For this review, use the dimensioned drawing (mm, ordinates from the lowest corner) and the shaded views. Coordinates: 2 decimals unless noted, no trailing zeros. Loops run counter-clockwise (first coordinate to the right, second up) from the corner with the lowest first, then second, coordinate; pieces in that order, holes last. Notation, with made-up numbers: (84, -2) - (95, -2) arc R19 cw to (95, 25) - close; hole circle Ø9 at (29, 16). An arc over 180 degrees is marked (long way). Return JSON: item names as keys, results as strings. Group by question number.
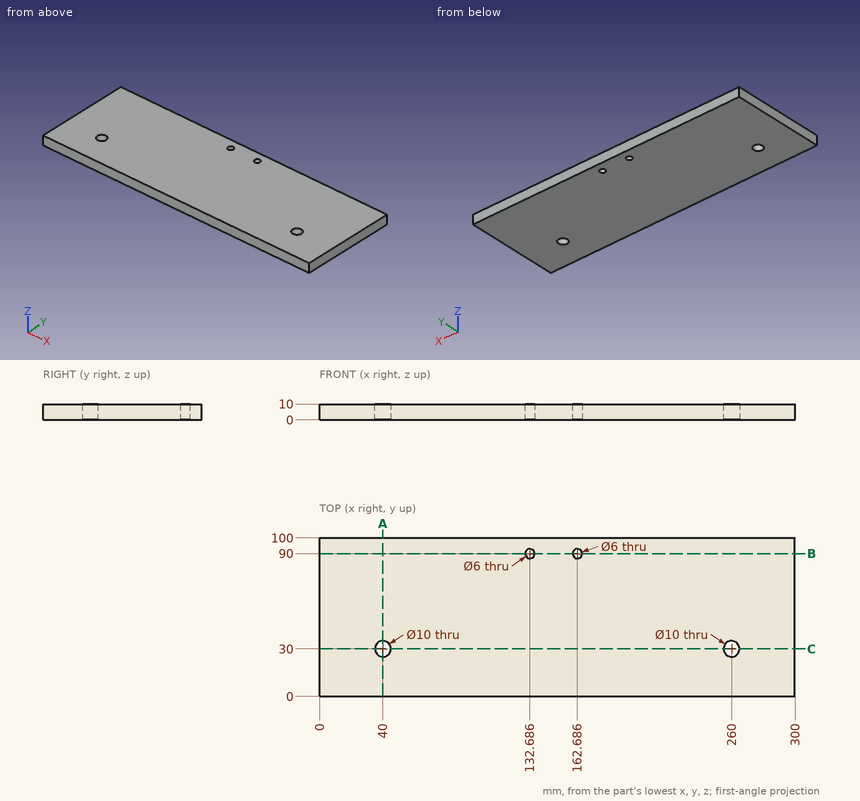
Item 1: Add section C-C (y = 30). State the section outline as (x, z) points, then the cut area to 3 significant figures.
Item 2: Add section A-A (x = 40). State the section outline as (y, z) points, then the cut area to 3 significant figures.
Item 3: To check wall thickness, follow line 1 (Y direction, x = 260, z = 4.75); line 2 (Y direction, x = 44, z = 8.25). State the ranges of each line that lie inside material, in increasing order. Write a range as from..to.
Item 4: Add section B-B (y = 90). State the section outline as (x, z) points, then the cut area to 3 significant figures.
Item 5: For P1, Ø8, axis at x = 40, y = 30, coming from the +Z side, flat-tipped, find the tip position at first contact; note if it passes through.
Answers below:
{
 "1": {"outline": "(0, 0) - (35, 0) - (35, 10) - (0, 10) - close; (45, 0) - (255, 0) - (255, 10) - (45, 10) - close; (265, 0) - (300, 0) - (300, 10) - (265, 10) - close", "area": "2,800 mm^2"},
 "2": {"outline": "(0, 0) - (25, 0) - (25, 10) - (0, 10) - close; (35, 0) - (100, 0) - (100, 10) - (35, 10) - close", "area": "900 mm^2"},
 "3": {"line 1": "y = 0..25, 35..100", "line 2": "y = 0..27, 33..100"},
 "4": {"outline": "(0, 0) - (129.69, 0) - (129.69, 10) - (0, 10) - close; (135.69, 0) - (159.69, 0) - (159.69, 10) - (135.69, 10) - close; (165.69, 0) - (300, 0) - (300, 10) - (165.69, 10) - close", "area": "2,880 mm^2"},
 "5": {"P1": "passes through"}
}
